Build history of the part. All positions in model axes, mm. A direction names the side the tool comes from. Give positions to 0.01 mm unless a question says otherwise; leave off trailing zeros. Order: outer loops, then holes, each group sorted by start corner. A loop starts at its lowest first (then second) coordinate and runs counter-clockwise, first axis right, second up. Notation, with made-up numbers: (-3.5, 87.25) - (11.5, 87.25) arc R8 cw to (11.5, 98.25) - close; hole circle Ø5 at (-13.5, -26.5). An arc over 180 degrees is marked (long way). Answer in a Markdown table with one row per item.
```python
from build123d import *

# Parameters (mm, degrees)
BOSS_EXTRU_1_DEPTH      = 108
ESQUISSE2_R             = 2.5
ESQUISSE2_R_2           = 4
ESQUISSE2_R_3           = 2
ENL_V_MAT_EXTRU_1_DEPTH = 109.455059817


with BuildPart() as part:
    # Esquisse1 → Boss.-Extru.1 (new, symmetric)
    with BuildSketch(Plane(origin=(0, 0, 0), x_dir=(0, 0, -1), z_dir=(1, 0, 0))):
        Polygon((-7.5, 6.5), (-7.5, -1), (7.5, -1), (7.5, 6.5), (6.5, 6.5), (6.5, 0), (-6.5, 0), (-6.5, 6.5), align=None)
    extrude(amount=BOSS_EXTRU_1_DEPTH, both=True)

    # Esquisse2 → Enlèv. mat.-Extru.1 (cut, through all)
    with BuildSketch(Plane(origin=(0, 0, 0), x_dir=(1, 0, 0), z_dir=(0, 1, 0))):
        with Locations(Location((-98, 0, 0), (0, 0, 270))):
            Circle(ESQUISSE2_R)
        with Locations(Location((49, 0, 0), (0, 0, 270))):
            Circle(ESQUISSE2_R_2)
        with Locations(Location((77, 0, 0), (0, 0, 270))):
            Circle(ESQUISSE2_R_3)
        with BuildLine():
            Line((95.570714214, 3.5), (95.570714214, -3.5))
            ThreePointArc((95.570714214, -3.5), (87, 0), (95.570714214, 3.5))
        make_face()
        Polygon((-8.175932032, 1.473487567), (-8.175932032, -1.501256313), (-2.970130241, -1.501256313), (-2.970130241, -3.267510492), (10.137334983, 0), (-2.970130241, 3.518623985), (-2.970130241, 1.473487567), align=None)
    extrude(amount=-ENL_V_MAT_EXTRU_1_DEPTH, mode=Mode.SUBTRACT)


solid = part.part
```
1. Cut at B-B on y = 4. Write the cut outline in (x, z), and give its area (3 significant figures).
Check result:
| item | result |
|---|---|
| outline | (-108, -7.5) - (108, -7.5) - (108, -6.5) - (-108, -6.5) - close; (-108, 6.5) - (108, 6.5) - (108, 7.5) - (-108, 7.5) - close |
| area | 432 mm² |
2. Cut at A-A on x = 92. Write the cut outline in (y, z), and give its area (3 significant figures).
Check result:
| item | result |
|---|---|
| outline | (-1, -7.5) - (6.5, -7.5) - (6.5, -6.5) - (0, -6.5) - (0, -5) - (-1, -5) - close; (-1, 5) - (0, 5) - (0, 6.5) - (6.5, 6.5) - (6.5, 7.5) - (-1, 7.5) - close |
| area | 18.0 mm² |
3. Drop flat-ended pins along their axis: P1, Ø4, axis at y = 4.5, z = -3.5, coming from the -X side; P2, Ø6, axis at x = -98, z = 0, coming from the +Y side. Give the stop position or say it passes through.
Check result:
| item | result |
|---|---|
| P1 | passes through |
| P2 | stops at y = 0 |
4. Probe line 1 (Z direction, x = 80, y = 1.75); line 2 (Y direction, x = 25.5, z = 3.5); line 3 (Z direction, x = 92, y = -0.25). List the from-to ranges inside material, lowest first.
Check result:
| item | result |
|---|---|
| line 1 | z = -7.5 to -6.5, 6.5 to 7.5 |
| line 2 | y = -1 to 0 |
| line 3 | z = -7.5 to -5, 5 to 7.5 |
5. Cut at C-C on x = -57. Write the cut outline in (y, z).
Check result:
| item | result |
|---|---|
| outline | (-1, -7.5) - (6.5, -7.5) - (6.5, -6.5) - (0, -6.5) - (0, 6.5) - (6.5, 6.5) - (6.5, 7.5) - (-1, 7.5) - close |
6. Two-plate mould, pull along Z, no slides. Class faces 3 (the face through (108, -0.3, 0)), 4 (the face through (2, 3, 6.5)), 5 (the face through (2, 3, -7.5)): +Z half, -Z half, draft (parallel to the pull), parting line (faces both ways), or undercut.
Check result:
| item | result |
|---|---|
| face 3 | draft |
| face 4 | undercut |
| face 5 | -Z half |
7. Which spindle directions (+Z, -Z, +X, -X, +Y, -Y) get a long thin tool onto all of the face, cutting with end or side? Do faces 1 (the face through (2, -1, 3)), 2 (the face through (2, 0, -3)). Say none if no direction does.
Check result:
| item | result |
|---|---|
| face 1 | +Z, -Z, +X, -X, -Y |
| face 2 | +X, -X, +Y |
8. Cut at D-D on x = 49. Write the cut outline in (y, z).
Check result:
| item | result |
|---|---|
| outline | (-1, -7.5) - (6.5, -7.5) - (6.5, -6.5) - (0, -6.5) - (0, -4) - (-1, -4) - close; (-1, 4) - (0, 4) - (0, 6.5) - (6.5, 6.5) - (6.5, 7.5) - (-1, 7.5) - close |
